```python
from build123d import *

# Parameters (mm, degrees)
BOSS_EXTRUDE1_DEPTH             = 100
M2X0_4_TAPPED_HOLE2_D           = 1.6
M2X0_4_TAPPED_HOLE2_CSINK_D     = 2.05
M2X0_4_TAPPED_HOLE2_CSINK_ANGLE = 90
LPATTERN1_COUNT                 = 3
LPATTERN1_PITCH                 = 35
M2X0_4_TAPPED_HOLE3_D           = 1.6
M2X0_4_TAPPED_HOLE3_CSINK_D     = 2.05
M2X0_4_TAPPED_HOLE3_CSINK_ANGLE = 90
LPATTERN2_COUNT                 = 3
LPATTERN2_PITCH                 = 35
M2X0_4_TAPPED_HOLE4_D           = 1.6
M2X0_4_TAPPED_HOLE4_CSINK_D     = 2.05
M2X0_4_TAPPED_HOLE4_CSINK_ANGLE = 90
M2X0_4_TAPPED_HOLE5_D           = 1.6
M2X0_4_TAPPED_HOLE5_CSINK_D     = 2.05
M2X0_4_TAPPED_HOLE5_CSINK_ANGLE = 90


with BuildPart() as part:
    # Sketch2 → Boss-Extrude1 (new body)
    with BuildSketch(Plane(origin=(0, 0, 0), x_dir=(1, 0, 0), z_dir=(0, 1, 0))):
        with BuildLine():
            Line((0, 0), (0, 7.5))
            ThreePointArc((0, 7.5), (0.292893219, 8.207106781), (1, 8.5))
            Line((1, 8.5), (8.5, 8.5))
            Line((8.5, 8.5), (8.5, 6))
            Line((8.5, 6), (2.5, 6))
            Line((2.5, 6), (2.5, 0))
            Line((2.5, 0), (0, 0))
        make_face()
    extrude(amount=BOSS_EXTRUDE1_DEPTH)

    # M2x0.4 Tapped Hole2 (through all)
    with Locations(Plane(origin=(0, 0, -8.5), x_dir=(-1, 0, 0), z_dir=(0, 0, -1))):
        with Locations((-4.25, 15)):
            m2x0_4_tapped_hole2 = CounterSinkHole(M2X0_4_TAPPED_HOLE2_D / 2, M2X0_4_TAPPED_HOLE2_CSINK_D / 2, counter_sink_angle=M2X0_4_TAPPED_HOLE2_CSINK_ANGLE)

    # LPattern1: M2x0.4 Tapped Hole2 ×3
    with Locations(*[(0, i * LPATTERN1_PITCH, 0) for i in range(1, LPATTERN1_COUNT)]):
        add(m2x0_4_tapped_hole2, mode=Mode.SUBTRACT)

    # M2x0.4 Tapped Hole3 (through all)
    with Locations(Plane.ZY):
        with Locations((-4.25, 15)):
            m2x0_4_tapped_hole3 = CounterSinkHole(M2X0_4_TAPPED_HOLE3_D / 2, M2X0_4_TAPPED_HOLE3_CSINK_D / 2, counter_sink_angle=M2X0_4_TAPPED_HOLE3_CSINK_ANGLE)

    # LPattern2: M2x0.4 Tapped Hole3 ×3
    with Locations(*[(0, i * LPATTERN2_PITCH, 0) for i in range(1, LPATTERN2_COUNT)]):
        add(m2x0_4_tapped_hole3, mode=Mode.SUBTRACT)

    # M2x0.4 Tapped Hole4 (through all)
    with Locations(Plane(origin=(0, 0, -8.5), x_dir=(-1, 0, 0), z_dir=(0, 0, -1))):
        with Locations((-4.25, 30)):
            CounterSinkHole(M2X0_4_TAPPED_HOLE4_D / 2, M2X0_4_TAPPED_HOLE4_CSINK_D / 2, counter_sink_angle=M2X0_4_TAPPED_HOLE4_CSINK_ANGLE)

    # M2x0.4 Tapped Hole5 (through all)
    with Locations(Plane.ZY):
        with Locations((-4.25, 30)):
            CounterSinkHole(M2X0_4_TAPPED_HOLE5_D / 2, M2X0_4_TAPPED_HOLE5_CSINK_D / 2, counter_sink_angle=M2X0_4_TAPPED_HOLE5_CSINK_ANGLE)


solid = part.part
```
Design review of the part built by this model. Coordinates are the model's own, in mm. A direction names the side the tool comes from. Round coordinates to 2 decimals unless told otherwise and drop trailing zeros. Write each loop counter-clockwise with the first axis right and the second up, starting at its lowest first coordinate (ties: lowest second). Pieces come first, ordered by that corner, then holes.
Item 1: For probe 1 along Y at (x, z) = (4.25, -7.7); probe 2 along X at (y, z) = (85, -6.9); probe 3 along Z at (x, y) = (0.95, 85), list the stretches that pass through material, from the lowest coordinate up.
Item 2: We need section B-B on z = -2. Write out the cut boundary in (x, y), and give its area (3 significant figures).
Item 3: For faces 1 (the flat face through (8.5, 49, -7)), 2 (the flat face through (2.5, 49, -3)), list the 3-axis set-ups (+Z, -Z, +X, -X, +Y, -Y) from which the entire face can be reached by the end or side of a thin tool; tool diameter is ignored.
Item 4: We need section A-A on y = 33.5. Write out the cut boundary in (x, z).
Item 5: Clearance check with flat-ended pins moving along their axes: pin 1 Ø1 at (y, z) = (53.5, -3.5) entering from +X; pin 2 Ø2 at (y, z) = (85, -4.25) entering from -X (3 decimals); pin 3 Ø1.4 at (y, z) = (50, -4.25) entering from -X; pin 4 Ø3 at (x, y) = (7, 29) entering from +Z. State where each tip first meets the part, or that it passes through.
Item 6: The part is to be moulded in two halves that separate along Z. For faces 3 (the cylindrical face through (4.146, 50.793, -7.122)), 4 (the cylindrical face through (1.38, 15.54, -3.66)), 5 (the flat face through (6, 49, -8.5)), 6 (the cylindrical face through (1.38, 84.22, -4.08)), say which applies: +Z half, -Z half, draft (parallel to the pull), parting line (faces both ways), or undercut.
Returned:
1. probe 1: y = 0 to 14.2, 15.8 to 29.2, 30.8 to 49.2, 50.8 to 84.2, 85.8 to 100
1. probe 2: x = 0 to 3.45, 5.05 to 8.5
1. probe 3: z = -8.5 to -5.05, -3.45 to 0
2. outline: (0, 0) - (2.5, 0) - (2.5, 100) - (0, 100) - close
2. area: 250 mm2
3. face 1: +Z, -Z, +X, +Y, -Y
3. face 2: +Z, +X, +Y, -Y
4. outline: (0, -7.5) arc R1 ccw to (1, -8.5) - (8.5, -8.5) - (8.5, -6) - (2.5, -6) - (2.5, 0) - (0, 0) - close
5. pin 1: stops at x = 2.5
5. pin 2: stops at x = 0.025
5. pin 3: passes through
5. pin 4: stops at z = -6
6. face 3: draft
6. face 4: undercut
6. face 5: -Z half
6. face 6: undercut
